Build history of the part. All positions in model axes, mm. A direction names the side the tool comes from. Give positions to 0.01 mm unless a question says otherwise; leave off trailing zeros. Write each loop counter-clockwise with the first axis right and the second up, starting at its lowest first coordinate (ties: lowest second). Pieces come first, ordered by that corner, then holes. Notation, with made-up numbers: (19.25, 1.25) -> (45.25, 1.25) arc R10 ccw to (45.25, 11.25) -> close; hole circle Ø1 at (80.25, -20.5). An arc over 180 degrees is marked (long way). Put each result on its own line as item: value.
Autodesk Inventor part; units mm, degrees
ref_plane "YZ Plane" through (0, 0, 0) normal (1, 0, 0) x (0, 1, 0)
ref_plane "XZ Plane" through (0, 0, 0) normal (0, 1, 0) x (-1, 0, 0)
ref_plane "XY Plane" through (0, 0, 0) normal (0, 0, 1) x (1, 0, 0)
sketch "Sketch1" plane through (0, 0, 0) normal (0, 1, 0) x (-1, 0, 0)
  circle A0 centre (26.0324, -0.4741) radius 1.5
  circle A1 centre (-24.2562, 0) radius 3
  circle A2 centre (-24.2562, 0) radius 1.5
  circle A3 centre (26.0324, -0.4741) radius 3
  line L0 (0, 0) -> (-28.1337, 0) construction
  line L1 (0, 0) -> (28.9947, 0) construction
  line L2 (28.9947, 0) -> (24.6719, 27.0084)
  line L3 (-23.6062, 24.8761) -> (-27.2238, 0.4393)
  line L4 (23.1627, -1.3485) -> (16.3374, 21.053)
  line L5 (16.3374, 21.053) -> (-19.0472, 21.053)
  line L6 (-19.0472, 21.053) -> (-21.2723, -0.3108)
  line L7 (24.6719, 27.0084) -> (-23.2906, 27.0084)
  line L8 (-23.2906, 27.0084) -> (-23.6062, 24.8761)
  dimension "d8" = 3
  dimension "d9" = 6
  dimension "d10" = 3
  dimension "d12" = 6
  dimension "d13" = 180
extrude "Extrusion1" add sketch "Sketch1" along normal blind 3
properties part number "barra_c"
1) Pull direction X, two halves, no side cores. Call faces 1 (the flat face through (-3, 3, 22)), 2 (the flat face through (-26.864, 1.479, 13.315)), 3 (the cylindrical face through (-26.77, 1.48, -3.38)): released by +X, released by -X, zero draft, split by the parting line, or undercut.
Filled sheet:
face 1: zero draft
face 2: released by -X
face 3: undercut
2) Slice it at B-B (y = 1.9). Write the cut outline in (x, z).
Filled sheet:
outline: (-28.99, 0) arc R3 ccw to (-23.16, -1.35) -> (-16.34, 21.05) -> (19.05, 21.05) -> (21.27, -0.31) arc R3 ccw (long way) to (27.22, 0.44) -> (23.61, 24.88) -> (23.29, 27.01) -> (-24.67, 27.01) -> close; hole circle Ø3 at (-26.03, -0.47); hole circle Ø3 at (24.26, 0)
3) Tool access for faces 4 (the flat face through (1, 1, 21.053)), 5 (the flat face through (-1, 1, 27.008)): list every direction of +Z, -Z, +X, -X, +Y, -Y with a clear straight run to the whole face (end or side of a thin tool).
Filled sheet:
face 4: -Z, +Y, -Y
face 5: +Z, +X, -X, +Y, -Y
4) Wall check: L1, parallel to X at y = 1.95, z = -1; L2, parallel to Z at x = -12, y = 0.35; L3, parallel to X at y = 2.8, z = 4.5. Give the ranges that are in metal, low to high.
Filled sheet:
L1: -28.99 to -27.44, -24.63 to -23.06, 21.43 to 23.14, 25.37 to 27.08
L2: 21.05 to 27.01
L3: -28.27 to -21.38, 20.77 to 26.62
5) Slice it at A-A (z = 4). Write the cut outline in (x, y).
Filled sheet:
outline: (-28.35, 0) -> (-21.53, 0) -> (-21.53, 3) -> (-28.35, 3) -> close; (20.82, 0) -> (26.7, 0) -> (26.7, 3) -> (20.82, 3) -> close
6) Slice it at C-C (z = 15). Write the cut outline in (x, y), plus the area to 3 significant figures.
Filled sheet:
outline: (-26.59, 0) -> (-18.18, 0) -> (-18.18, 3) -> (-26.59, 3) -> close; (19.68, 0) -> (25.07, 0) -> (25.07, 3) -> (19.68, 3) -> close
area: 41.4 mm2
7) Slice it at D-D (x = 10.5). Write the cut outline in (y, z), plus the area to 3 significant figures.
Filled sheet:
outline: (0, 21.05) -> (3, 21.05) -> (3, 27.01) -> (0, 27.01) -> close
area: 17.9 mm2
8) Pin check, flat tips, straight feed: pin 1 (1.5 mm diameter, centred on x = -4, y = 2, fed in from -Z); pin 2 (3.5 mm diameter, centred on x = 24.26, z = 0, fed in from +Y). Stop position of each tip, or through.
Filled sheet:
pin 1: z = 21.05
pin 2: y = 3
